```python
from build123d import *

# Parameters (mm, degrees)
SKETCH2_W           = 93.5
SKETCH2_H           = 56
BOSS_EXTRUDE1_DEPTH = 3
SKETCH3_R           = 1.5
CUT_EXTRUDE5_DEPTH  = 4
SKETCH5_R           = 3.025
CUT_EXTRUDE7_DEPTH  = 2.5
SKETCH6_W           = 2.5
SKETCH6_H           = 2.5
SKETCH6_W_2         = 6.5
SKETCH6_H_2         = 8.5
SKETCH6_W_3         = 21
SKETCH6_H_3         = 11
BOSS_EXTRUDE2_DEPTH = 35
SKETCH8_R           = 1.5
CUT_EXTRUDE8_DEPTH  = 4
SKETCH9_W           = 10
SKETCH9_H           = 2
CUT_EXTRUDE9_DEPTH  = 1.5
SKETCH11_W          = 2.5
SKETCH11_H          = 29
BOSS_EXTRUDE4_DEPTH = 10
SKETCH12_W          = 2.5
SKETCH12_H          = 29
BOSS_EXTRUDE5_DEPTH = 4


with BuildPart() as part:
    # Sketch2 → Boss-Extrude1 (new body)
    with BuildSketch(Plane(origin=(0, 0, 0), x_dir=(1, 0, 0), z_dir=(0, 1, 0))):
        with Locations((-29.736211897, 0.601935214)):
            Rectangle(SKETCH2_W, SKETCH2_H)
    extrude(amount=BOSS_EXTRUDE1_DEPTH)

    # Sketch3 → Cut-Extrude5 (cut, through all)
    with BuildSketch(Plane(origin=(0, 3, 0), x_dir=(1, 0, 0), z_dir=(0, 1, 0))):
        with Locations((-13.486211897, 12.601935214)):
            Circle(SKETCH3_R)
        with Locations((-13.486211897, -11.398064786)):
            Circle(SKETCH3_R)
        with Locations((-71.986211897, 0.601935214)):
            Circle(SKETCH3_R)
    extrude(amount=-CUT_EXTRUDE5_DEPTH, mode=Mode.SUBTRACT)

    # Sketch5 → Cut-Extrude7 (cut)
    with BuildSketch(Plane(origin=(0, 0, 0), x_dir=(-1, 0, 0), z_dir=(0, -1, 0))):
        with Locations((26.486211897, 15.851935214)):
            Circle(SKETCH5_R)
        with Locations((26.486211897, -14.648064786)):
            Circle(SKETCH5_R)
        with Locations((56.986211897, -14.648064786)):
            Circle(SKETCH5_R)
        with Locations((56.986211897, 15.851935214)):
            Circle(SKETCH5_R)
    extrude(amount=-CUT_EXTRUDE7_DEPTH, mode=Mode.SUBTRACT)

    # Sketch6 → Boss-Extrude2 (add)
    with BuildSketch(Plane(origin=(0, 3, 0), x_dir=(1, 0, 0), z_dir=(0, 1, 0))):
        with Locations((15.763788103, 27.351935214)):
            Rectangle(SKETCH6_W, SKETCH6_H)
        with Locations((11.263788103, 27.351935214)):
            Rectangle(SKETCH6_W_2, SKETCH6_H)
        with Locations((15.763788103, 21.851935214)):
            Rectangle(SKETCH6_W, SKETCH6_H_2)
        Polygon((17.013788103, -11.398064786), (14.513788103, -11.398064786), (14.513788103, -24.898064786), (14.513788103, -27.398064786), (17.013788103, -27.398064786), align=None)
        with Locations((4.013788103, -26.148064786)):
            Rectangle(SKETCH6_W_3, SKETCH6_H)
        with Locations((-75.236211897, -19.398064786)):
            Rectangle(SKETCH6_W, SKETCH6_H_3)
        Polygon((-73.986211897, -24.898064786), (-76.486211897, -24.898064786), (-76.486211897, -27.398064786), (-54.486211897, -27.398064786), (-54.486211897, -24.898064786), align=None)
        Polygon((-76.486211897, 28.601935214), (-76.486211897, 26.101935214), (-73.986211897, 26.101935214), (-67.486211897, 26.101935214), (-67.486211897, 28.601935214), align=None)
        with Locations((-75.236211897, 20.601935214)):
            Rectangle(SKETCH6_W, SKETCH6_H_3)
    extrude(amount=BOSS_EXTRUDE2_DEPTH)

    # Sketch8 → Cut-Extrude8 (cut, through all)
    with BuildSketch(Plane(origin=(0, 3, 0), x_dir=(1, 0, 0), z_dir=(0, 1, 0))):
        with Locations((-69.486211897, -20.398064786)):
            Circle(SKETCH8_R)
        with Locations((-69.486211897, 21.601935214)):
            Circle(SKETCH8_R)
        with Locations((9.513788103, -20.398064786)):
            Circle(SKETCH8_R)
        with Locations((9.513788103, 21.601935214)):
            Circle(SKETCH8_R)
    extrude(amount=-CUT_EXTRUDE8_DEPTH, mode=Mode.SUBTRACT)

    # Sketch9 → Cut-Extrude9 (cut)
    with BuildSketch(Plane(origin=(0, 0, 0), x_dir=(-1, 0, 0), z_dir=(0, -1, 0))):
        with Locations((68.486211897, 27.601935214)):
            Rectangle(SKETCH9_W, SKETCH9_H)
        with Locations((68.486211897, -26.398064786)):
            Rectangle(SKETCH9_W, SKETCH9_H)
        with Locations((14.486211897, 27.601935214)):
            Rectangle(SKETCH9_W, SKETCH9_H)
        with Locations((14.486211897, -26.398064786)):
            Rectangle(SKETCH9_W, SKETCH9_H)
    extrude(amount=-CUT_EXTRUDE9_DEPTH, mode=Mode.SUBTRACT)

    # Sketch11 → Boss-Extrude4 (add)
    with BuildSketch(Plane(origin=(0, 3, 0), x_dir=(1, 0, 0), z_dir=(0, 1, 0))):
        with Locations((15.763788103, 3.101935214)):
            Rectangle(SKETCH11_W, SKETCH11_H)
    extrude(amount=BOSS_EXTRUDE4_DEPTH)

    # Sketch12 → Boss-Extrude5 (add)
    with BuildSketch(Plane(origin=(0, 3, 0), x_dir=(1, 0, 0), z_dir=(0, 1, 0))):
        with Locations((-75.236211897, 0.601935214)):
            Rectangle(SKETCH12_W, SKETCH12_H)
    extrude(amount=BOSS_EXTRUDE5_DEPTH)


solid = part.part
```
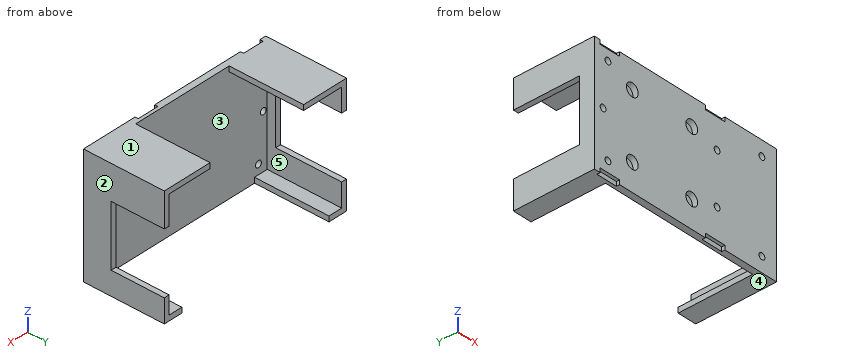
Design review of the part built by this model. Coordinates are the model's own, in mm. Face numbers are marked on the shaded views. A direction names the side the tool comes from. Coordinates: 2 decimals unless noted, no trailing zeros. Order: outer loops, then holes, each group sorted by start corner. A loop starts at its lowest first (then second) coordinate and runs counter-clockwise, first axis right, second up. Notation, with made-up numbers: (48.25, -14.75) - (94.25, -14.75) arc R32 ccw to (94.25, 13.25) - close; hole circle Ø9 at (50, -30). An arc over 180 degrees is marked (long way). Answer in a Markdown table with one row per item.
(1) Consider section A-A on y = 12. State the section outline as (x, z) points, plus the area to 3 significant figures.
Checked values:
| item | result |
|---|---|
| outline | (-76.49, -28.6) - (-67.49, -28.6) - (-67.49, -26.1) - (-73.99, -26.1) - (-73.99, -15.1) - (-76.49, -15.1) - close; (-76.49, 13.9) - (-73.99, 13.9) - (-73.99, 24.9) - (-54.49, 24.9) - (-54.49, 27.4) - (-76.49, 27.4) - close; (-6.49, 24.9) - (14.51, 24.9) - (14.51, -26.1) - (8.01, -26.1) - (8.01, -28.6) - (17.01, -28.6) - (17.01, 27.4) - (-6.49, 27.4) - close |
| area | 341 mm^2 |
(2) For the marked faces 4 and 5, list the 3-axis set-ups (+Z, -Z, +X, -X, +Y, -Y) from which the entire face can be reached by the end or side of a thin tool; tool diameter is ignored.
Checked values:
| item | result |
|---|---|
| face 4 | -Z, +X, -X, +Y, -Y |
| face 5 | +Y |
(3) Consider section C-C on x = -8.5. State the section outline as (y, z) points.
Checked values:
| item | result |
|---|---|
| outline | (0, -28.6) - (3, -28.6) - (3, 27.4) - (0, 27.4) - close |
(4) Consider section D-D on z = -24.5. State the section outline as (x, y) points.
Checked values:
| item | result |
|---|---|
| outline | (-76.49, 0) - (17.01, 0) - (17.01, 38) - (14.51, 38) - (14.51, 3) - (-73.99, 3) - (-73.99, 38) - (-76.49, 38) - close |
(5) The part is to be moulded in two halves that separate along X. For the marked faces 1, 2 and 3, say which applies: released by +X, released by -X, zero draft, split by the parting line, or undercut.
Checked values:
| item | result |
|---|---|
| face 1 | zero draft |
| face 2 | released by +X |
| face 3 | undercut |
(6) Consider section B-B on z = 7.5. State the section outline as (x, y) points, plus the area to 4 significant figures.
Checked values:
| item | result |
|---|---|
| outline | (-76.49, 0) - (17.01, 0) - (17.01, 13) - (14.51, 13) - (14.51, 3) - (-73.99, 3) - (-73.99, 7) - (-76.49, 7) - close |
| area | 315.5 mm^2 |
(7) Clearance check with flat-ended pins moving along their axes: pin 1 (12 mm diameter, centred on y = 11, z = -5.5, fed in from -X); pin 2 (12 mm diameter, centred on x = -28.5, z = -0.5, fed in from +Y); pin 3 (12 mm diameter, centred on x = -5, y = 33.5, fed in from -Z); pin 4 (1.8 mm diameter, centred on x = 9.51, z = 20.4, fed in from -Y). State where each tip first meets the part, or that it passes through.
Checked values:
| item | result |
|---|---|
| pin 1 | x = -76.49 |
| pin 2 | y = 3 |
| pin 3 | z = 24.9 |
| pin 4 | through |
(8) Wall thickness on line 1 along X through (y, z) = (32, -25.5); line 2 along Z through (x, y) = (-69, 6); line 3 along Y through (x, z) = (-21, -21): over which ranges is each line inside the solid? List them lowest first. Write a range as from..to.
Checked values:
| item | result |
|---|---|
| line 1 | -76.49..-73.99, 14.51..17.01 |
| line 2 | -28.6..-26.1, 24.9..27.4 |
| line 3 | 0..3 |
